from build123d import *

# Parameters (mm, degrees)
SKETCH038_R           = 18.65
SKETCH038_R_2         = 6.05
PAD010_DEPTH          = 5.5
SKETCH039_R           = 3.6
SKETCH039_R_2         = 1.25
POCKET008_DEPTH       = 111.57324
POLARPATTERN001_COUNT = 5


with BuildPart() as part:
    # Sketch038 → Pad010 (new body)
    with BuildSketch(Plane.XY):
        Circle(SKETCH038_R)
        Circle(SKETCH038_R_2, mode=Mode.SUBTRACT)
    extrude(amount=PAD010_DEPTH)

    # Sketch039 → Pocket008 (cut, through all)
    with BuildSketch(Plane.XY):
        with Locations((12.45, 0)):
            Circle(SKETCH039_R)
        with Locations((10.881279, 7.905712)):
            Circle(SKETCH039_R_2)
    pocket008 = extrude(amount=POCKET008_DEPTH, mode=Mode.SUBTRACT)

    # PolarPattern001: Pocket008 ×5 about axis
    polarpattern001_axis = Axis((0, 0, 0), (0, 0, 1))
    for i in range(1, POLARPATTERN001_COUNT):
        add(pocket008.rotate(polarpattern001_axis, i * 360 / POLARPATTERN001_COUNT), mode=Mode.SUBTRACT)


with BuildPart() as part_1:
    # Body009 placement: moved
    add(part.part.moved(Location((0, 0, 15))))


solid = part_1.part
Build history of the part. All positions in model axes, mm. Give positions to 0.01 mm unless a question says otherwise; leave off trailing zeros. Loops run counter-clockwise (first coordinate to the right, second up) from the corner with the lowest first, then second, coordinate; pieces in that order, holes last. Notation, with made-up numbers: (84.25, 51) -> (105.25, 51) arc R18 cw to (105.25, 62) -> close; hole circle Ø2 at (7, -19). An arc over 180 degrees is marked (long way). Answer in a Markdown table with one row per item.
Item 1: Flat gauge pins, fed straight in: P1, Ø1.5, axis at x = -7.5, z = 18, coming from the -Y side; P2, Ø1.5, axis at x = -4.16, y = -12.79, coming from the -Z side; P3, Ø2, axis at x = 5, z = 16, coming from the +Y side; P4, Ø2, axis at x = 5.5, z = 18, coming from the -Y side. Where does each tip first touch, or does it go through?
Findings below:
| item | result |
|---|---|
| P1 | stops at y = -17.39 |
| P2 | passes through |
| P3 | stops at y = 18.22 |
| P4 | stops at y = -18.1 |
Item 2: Probe line 1 along Y through (x, z) = (0, 18.5); line 2 along Y through (x, z) = (-10, 19.8); line 3 along X through (y, z) = (12, 17.4). List the from-to ranges inside material, lowest first. Write a range as [from, to].
Findings below:
| item | result |
|---|---|
| line 1 | y = [-18.65, -6.05], [6.05, 18.65] |
| line 2 | y = [-15.74, -10.92], [-3.72, 3.72], [10.92, 15.74] |
| line 3 | x = [-14.28, -5.12], [-3.19, 0.25], [7.44, 14.28] |
Item 3: Mould opens along Y. For faces 1 (the cylindrical face through (-4.951, 13.757, 17.712)), 2 (the cylindrical face through (2.585, 8.469, 17.712)), 3 (the flat face through (8, 0, 20.5)), 4 (the cylindrical face through (-14.8, -11.35, 17.71)) say: pulls with the +Y half, pulls with the -Y half, needs draft (parallel to the pull), parting line crosses it, or undercut.
Findings below:
| item | result |
|---|---|
| face 1 | undercut |
| face 2 | undercut |
| face 3 | needs draft |
| face 4 | parting line crosses it |
Item 4: Slice it at B-B on x = -1.5. Write the cut outline in (y, z).
Findings below:
| item | result |
|---|---|
| outline | (-18.59, 15) -> (-5.86, 15) -> (-5.86, 20.5) -> (-18.59, 20.5) -> close; (5.86, 15) -> (18.59, 15) -> (18.59, 20.5) -> (5.86, 20.5) -> close |
Item 5: Slice it at D-D on z = 19.6. Give the number of separate pieces and of enclosed holes in the cut face, plus the area to 3 significant figures.
Findings below:
| item | result |
|---|---|
| separate pieces | 1 |
| enclosed holes | 11 |
| area | 750 mm² |
Item 6: Slice it at C-C on x = 6.5. Write the cut outline in (y, z), plus the area to 3 significant figures.
Findings below:
| item | result |
|---|---|
| outline | (-17.48, 15) -> (-14.27, 15) -> (-14.27, 20.5) -> (-17.48, 20.5) -> close; (-9.41, 15) -> (9.41, 15) -> (9.41, 20.5) -> (-9.41, 20.5) -> close; (14.27, 15) -> (17.48, 15) -> (17.48, 20.5) -> (14.27, 20.5) -> close |
| area | 139 mm² |
Item 7: Slice it at A-A on y = 0. Write the cut outline in (x, z).
Findings below:
| item | result |
|---|---|
| outline | (-18.65, 15) -> (-14.7, 15) -> (-14.7, 20.5) -> (-18.65, 20.5) -> close; (-12.2, 15) -> (-6.05, 15) -> (-6.05, 20.5) -> (-12.2, 20.5) -> close; (6.05, 15) -> (8.85, 15) -> (8.85, 20.5) -> (6.05, 20.5) -> close; (16.05, 15) -> (18.65, 15) -> (18.65, 20.5) -> (16.05, 20.5) -> close |
